from build123d import *

# Parameters (mm, degrees)
SKETCH_1_W            = 40
SKETCH_1_H            = 39
EXTRUDE_1_DEPTH       = 20
SKETCH_4_W            = 20
SKETCH_4_H            = 3.215179838
EXTRUDE_2_DEPTH       = 5
SKETCH_5_W            = 20
SKETCH_5_H            = 3.215179838
EXTRUDE_3_DEPTH       = 5
SKETCH_7_R            = 2
CUT_EXTRUDE_2_DEPTH   = 3.21517984
SKETCH_8_R            = 2
CUT_EXTRUDE_3_DEPTH   = 3.21517984
EXTRUDE_7_DEPTH       = 1
EXTRUDE_7_DEPTH_BACK  = 39
SKETCH_9_R            = 6
EXTRUDE_9_DEPTH       = 1
EXTRUDE_9_DEPTH_BACK  = 40
SKETCH_10_R           = 5
EXTRUDE_10_DEPTH      = 3
EXTRUDE_10_DEPTH_BACK = 41
SKETCH_11_R           = 3
SKETCH_12_R           = 0.705262345
CUT_EXTRUDE_4_DEPTH   = 40


with BuildPart() as part:
    # 草图1 → 凸台-拉伸1 (new body)
    with BuildSketch(Plane.XY):
        with Locations((-12.988047809, 18.294260929)):
            Rectangle(SKETCH_1_W, SKETCH_1_H)
    extrude(amount=EXTRUDE_1_DEPTH)

    # 草图4 → 凸台-拉伸2 (add)
    with BuildSketch(Plane.ZY.offset(32.988047809)):
        with Locations((10, 28.18667101)):
            Rectangle(SKETCH_4_W, SKETCH_4_H)
    extrude(amount=EXTRUDE_2_DEPTH)

    # 草图5 → 凸台-拉伸3 (add)
    with BuildSketch(Plane(origin=(7.011952191, 0, 0), x_dir=(0, 0, -1), z_dir=(1, 0, 0))):
        with Locations((-10, 28.18667101)):
            Rectangle(SKETCH_5_W, SKETCH_5_H)
    extrude(amount=EXTRUDE_3_DEPTH)

    # 草图7 → 切除-拉伸2 (cut)
    with BuildSketch(Plane(origin=(0, 29.794260929, 0), x_dir=(1, 0, 0), z_dir=(0, 1, 0))):
        with Locations(Location((-35.488047809, -5.338978439, 0), (0, 0, 270))):
            Circle(SKETCH_7_R)
        with Locations(Location((-35.488047809, -14.731505131, 0), (0, 0, 270))):
            Circle(SKETCH_7_R)
    extrude(amount=-CUT_EXTRUDE_2_DEPTH, mode=Mode.SUBTRACT)

    # 草图8 → 切除-拉伸3 (cut)
    with BuildSketch(Plane(origin=(0, 29.794260929, 0), x_dir=(1, 0, 0), z_dir=(0, 1, 0))):
        with Locations(Location((9.511952191, -5, 0), (0, 0, 270))):
            Circle(SKETCH_8_R)
        with Locations(Location((9.511952191, -15, 0), (0, 0, 270))):
            Circle(SKETCH_8_R)
    extrude(amount=-CUT_EXTRUDE_3_DEPTH, mode=Mode.SUBTRACT)

    # 草图9 → 凸台-拉伸7 (add, two sides: drawn at the far end of the back side and taken through both)
    with BuildSketch(Plane(origin=(0, 37.794260929, 0), x_dir=(1, 0, 0), z_dir=(0, 1, 0)).offset(-EXTRUDE_7_DEPTH_BACK)):
        with Locations(Location((-25.244994163, -10, 0), (0, 0, 90))):
            Circle(SKETCH_9_R)
    extrude(amount=EXTRUDE_7_DEPTH + EXTRUDE_7_DEPTH_BACK)

    # 草图10 → 凸台-拉伸9 (add, two sides: drawn at the far end of the back side and taken through both)
    with BuildSketch(Plane(origin=(0, 38.794260929, 0), x_dir=(1, 0, 0), z_dir=(0, 1, 0)).offset(-EXTRUDE_9_DEPTH_BACK)):
        with Locations(Location((-25.244994163, -10, 0), (0, 0, 270))):
            Circle(SKETCH_10_R)
    extrude(amount=EXTRUDE_9_DEPTH + EXTRUDE_9_DEPTH_BACK)

    # 草图11 → 凸台-拉伸10 (add, two sides: drawn at the far end of the back side and taken through both)
    with BuildSketch(Plane(origin=(0, 39.794260929, 0), x_dir=(1, 0, 0), z_dir=(0, 1, 0)).offset(-EXTRUDE_10_DEPTH_BACK)):
        with Locations(Location((-25.244994163, -10, 0), (0, 0, 270))):
            Circle(SKETCH_11_R)
    extrude(amount=EXTRUDE_10_DEPTH + EXTRUDE_10_DEPTH_BACK)

    # 草图12 → 切除-拉伸4 (cut)
    with BuildSketch(Plane(origin=(0, 42.794260929, 0), x_dir=(1, 0, 0), z_dir=(0, 1, 0))):
        with Locations(Location((-25.244994163, -10, 0), (0, 0, 270))):
            Circle(SKETCH_12_R)
    extrude(amount=-CUT_EXTRUDE_4_DEPTH, mode=Mode.SUBTRACT)


solid = part.part
Verification items for the finished model (mm, model axes). A direction names the side the tool comes from. Give positions to 0.01 mm unless a question says otherwise; leave off trailing zeros. Order: outer loops, then holes, each group sorted by start corner. A loop starts at its lowest first (then second) coordinate and runs counter-clockwise, first axis right, second up. Notation, with made-up numbers: M 80.5,81.5 L 88.5,81.5 A24 cw 88.5,106.5 Z; hole C 4.25,-22.5 d9. An arc over 180 degrees is marked long. Answer as a JSON object with one key per item and string values. Group by question number.
1) Cross-section at A-A (z = 1.5). Enter the section's corners in (x, y).
2) Mould release check, pull along X, two halves, no side actions. Record for faces 1 (the face through (-25.674, 23.074, 9.44)), 2 (the face through (-32.988, 34, 10)), 3 (the face through (-26.394, 41.273, 12.771)), 4 (the face through (-35, 26.579, 10)): released by +X, released by -X, zero draft, split by the parting line, or undercut.
3) Scan lines: line 1 along X through (y, z) = (35, 10); line 2 along X through (y, z) = (28.7, 15); line 3 along X through (y, z) = (29, 10). Record each from-to range of solid material in increasing order. Write a range as [from, to].
4) Access from +Z, -Z, +X, -X, +Y, -Y to the whole of each face (thin tool, end or side, straight path). Record for faces 5 (the face through (-25, 2.794, 10)), 6 (the face through (-32.988, 12, 10)), 7 (the face through (9, 26.579, 10)), 8 (the face through (9, 29.794, 10)).
5) Depth check by flat-ended pin: pin 1 Ø4.5 at (x, z) = (9.51, 15) entering from +Y; pin 2 Ø1 at (x, z) = (6.5, 17) entering from +Y; pin 3 Ø1.5 at (x, z) = (10, 9.5) entering from -Y. Enter the tip coordinate at first touch or a pass-through.
6) Cross-section at C-C (y = 23). Enter the section's corners in (x, z) (3 decimals), then the cut area to 3 significant figures.
7) Cross-section at B-B (z = 10). Enter the section's corners in (x, y) (3 decimals), then the cut area to 3 significant figures.
Result sheet:
{
 "1": {"outline": "M -37.99,26.58 L -32.99,26.58 L -32.99,-1.21 L 7.01,-1.21 L 7.01,26.58 L 12.01,26.58 L 12.01,29.79 L 7.01,29.79 L 7.01,37.79 L -32.99,37.79 L -32.99,29.79 L -37.99,29.79 Z"},
 "2": {"face 1": "undercut", "face 2": "released by -X", "face 3": "split by the parting line", "face 4": "zero draft"},
 "3": {"line 1": "x = [-32.99, -25.95], [-24.54, 7.01]", "line 2": "x = [-37.99, -37.47], [-33.51, 7.51], [11.51, 12.01]", "line 3": "x = [-37.99, -25.95], [-24.54, 12.01]"},
 "4": {"face 5": "+Y", "face 6": "+Z, -Z, -X, -Y", "face 7": "+Z, -Z, +X, -Y", "face 8": "+Z, -Z, +X, +Y"},
 "5": {"pin 1": "stops at y = 29.79", "pin 2": "stops at y = 37.79", "pin 3": "stops at y = 26.58"},
 "6": {"outline": "M -32.988,0 L 7.012,0 L 7.012,20 L -32.988,20 Z; hole C -25.245,10 d1.411", "area": "798 mm2"},
 "7": {"outline": "M -37.988,26.579 L -32.988,26.579 L -32.988,-1.206 L 7.012,-1.206 L 7.012,26.579 L 12.012,26.579 L 12.012,29.794 L 7.012,29.794 L 7.012,37.794 L -19.245,37.794 L -19.245,38.794 L -20.245,38.794 L -20.245,39.794 L -22.245,39.794 L -22.245,42.794 L -24.54,42.794 L -24.54,2.794 L -25.95,2.794 L -25.95,42.794 L -28.245,42.794 L -28.245,39.794 L -30.245,39.794 L -30.245,38.794 L -31.245,38.794 L -31.245,37.794 L -32.988,37.794 L -32.988,29.794 L -37.988,29.794 Z", "area": "1,580 mm2"}
}
